Part print with two shaded views. Sizes in mm from the minimum x, y, z corner. Coordinates: 2 decimals unless noted, no trailing zeros. Loops run counter-clockwise (first coordinate to the right, second up) from the corner with the lowest first, then second, coordinate; pieces in that order, holes last. Notation, with made-up numbers: (0.25, 63) -> (23.25, 63) arc R24 cw to (23.25, 94) -> close; hole circle Ø9 at (-1, 22.5). An arc over 180 degrees is marked (long way). Answer as a JSON object with one key per item and string values. Group by question number.
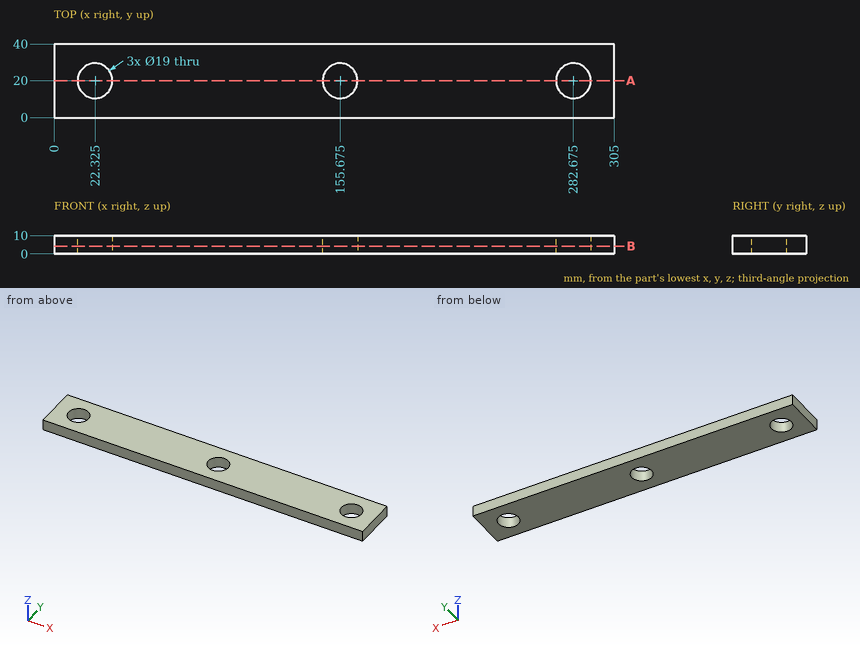
Item 1: Band-saw the part on A-A, the plane y = 20. List the corners of the cut face in (x, z) (3 decimals), and give its area (3 significant figures).
Item 2: Drill centre lines: L1, parallel to Y at x = 155.5, z = 4.5; L2, parallel to X at y = 15, z = 9; L3, parallel to X at y = 23, z = 6.5. Where is each one in solid material? Low to high.
Item 3: Band-saw the part on B-B, the plane z = 4.25. List the corners of the cut face in (x, y) (3 decimals), and give its area (3 significant figures).
Reply:
{
 "1": {"outline": "(0, 0) -> (12.825, 0) -> (12.825, 10) -> (0, 10) -> close; (31.825, 0) -> (146.175, 0) -> (146.175, 10) -> (31.825, 10) -> close; (165.175, 0) -> (273.175, 0) -> (273.175, 10) -> (165.175, 10) -> close; (292.175, 0) -> (305, 0) -> (305, 10) -> (292.175, 10) -> close", "area": "2,480 mm²"},
 "2": {"L1": "0 to 10.5, 29.5 to 40", "L2": "0 to 14.25, 30.4 to 147.6, 163.75 to 274.6, 290.75 to 305", "L3": "0 to 13.31, 31.34 to 146.66, 164.69 to 273.66, 291.69 to 305"},
 "3": {"outline": "(0, 0) -> (305, 0) -> (305, 40) -> (0, 40) -> close; hole circle Ø19 at (22.325, 20); hole circle Ø19 at (155.675, 20); hole circle Ø19 at (282.675, 20)", "area": "11,300 mm²"}
}
